For this review, take the finished solid that the model builds, in its own axes (mm). Coordinates: 2 decimals unless noted, no trailing zeros. Loops run counter-clockwise (first coordinate to the right, second up) from the corner with the lowest first, then second, coordinate; pieces in that order, holes last. Notation, with made-up numbers: M 58.25,61 L 98.25,61 A8 cw 98.25,74 Z; hole C 51,22.5 d9. An arc over 180 degrees is marked long. Answer as a JSON object with one key per item and string values. Group by question number.
Item 1: Add section B-B (y = 0). State the section outline as (x, z) points.
Item 2: Insertion check: pin 1 (2.5 mm diameter, centred on x = 3, y = -2, fed in from -Z). The pin has a flat end and moves straight along its axis. Give the tip position at first contact, or say it passes through.
Item 3: Add section A-A (x = 0). State the section outline as (y, z) points.
Item 4: Wall thickness on L1, parallel to Z at x = 4, y = -3.5: over which ranges is the line inside the solid? List them lowest first. Write a range as from..to.
Item 5: Add section C-C (y = -2.5). State the section outline as (x, z) points, then the cut area to 3 significant figures.
from build123d import *

# Parameters (mm, degrees)
SKETCH_W     = 8
SKETCH_H     = 8
PAD_DEPTH    = 9.6
FILLET_R     = 0.2
SKETCH001_R  = 0.25
PAD001_DEPTH = 3.5


with BuildPart() as fillet_body:
    # Sketch → Pad (new body)
    with BuildSketch(Plane.XY.offset(0.1)):
        with Locations((2.5, 0)):
            Rectangle(SKETCH_W, SKETCH_H)
    extrude(amount=PAD_DEPTH)

    # Fillet
    fillet_edges = [fillet_body.edges().sort_by_distance(p)[0] for p in [
        (6.5, -4, 4.9),
        (6.5, 4, 4.9),
        (-1.5, -4, 4.9),
        (-1.5, 4, 4.9),
    ]]
    fillet(fillet_edges, radius=FILLET_R)


with BuildPart() as obj1:
    # Sketch001 → Pad001 (new body)
    with BuildSketch(Plane.XY.offset(0.5)):
        Circle(SKETCH001_R)
        with Locations((5, 0)):
            Circle(SKETCH001_R)
    extrude(amount=-PAD001_DEPTH)

    # obj1: union Fillet body
    add(fillet_body.part)


solid = obj1.part
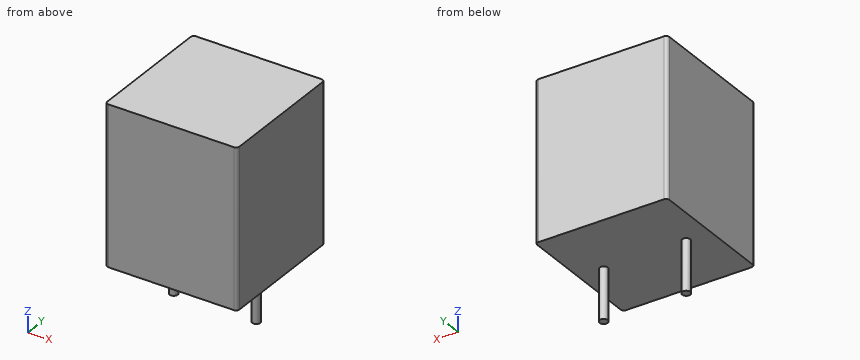
From the geometry:
{
 "1": {"outline": "M -1.5,0.1 L -0.25,0.1 L -0.25,-3 L 0.25,-3 L 0.25,0.1 L 4.75,0.1 L 4.75,-3 L 5.25,-3 L 5.25,0.1 L 6.5,0.1 L 6.5,9.7 L -1.5,9.7 Z"},
 "2": {"pin 1": "stops at z = 0.1"},
 "3": {"outline": "M -4,0.1 L -0.25,0.1 L -0.25,-3 L 0.25,-3 L 0.25,0.1 L 4,0.1 L 4,9.7 L -4,9.7 Z"},
 "4": {"L1": "z = 0.1..9.7"},
 "5": {"outline": "M -1.5,0.1 L 6.5,0.1 L 6.5,9.7 L -1.5,9.7 Z", "area": "76.8 mm²"}
}
